```python
from build123d import *

# Parameters (mm, degrees)
BOSS_EXTRUDE2_DEPTH = 6.35
SKETCH4_R           = 1.5
CUT_EXTRUDE1_DEPTH  = 6.35
SKETCH5_R           = 1.25
SKETCH5_W           = 6.35
SKETCH5_H           = 19.05
CUT_EXTRUDE2_DEPTH  = 6.35
SKETCH6_R           = 1.5
CUT_EXTRUDE3_DEPTH  = 6.35
SKETCH7_R           = 1.5
SKETCH7_W           = 6.35
SKETCH7_H           = 19.05
CUT_EXTRUDE4_DEPTH  = 6.35
SKETCH9_R           = 1.5
CUT_EXTRUDE6_DEPTH  = 6.35
SKETCH10_R          = 1.5
CUT_EXTRUDE7_DEPTH  = 7.35


with BuildPart() as part:
    # Sketch3 → Boss-Extrude2 (new body)
    with BuildSketch(Plane(origin=(0, 0, 0), x_dir=(1, 0, 0), z_dir=(0, 1, 0))):
        with BuildLine():
            Line((-156.21, -76.2), (156.21, -76.2))
            ThreePointArc((156.21, -76.2), (174.170512242, -68.760512242), (181.61, -50.8))
            Line((181.61, -50.8), (181.61, 50.8))
            ThreePointArc((181.61, 50.8), (174.170512242, 68.760512242), (156.21, 76.2))
            Line((156.21, 76.2), (-156.21, 76.2))
            ThreePointArc((-156.21, 76.2), (-174.170512242, 68.760512242), (-181.61, 50.8))
            Line((-181.61, 50.8), (-181.61, -50.8))
            ThreePointArc((-181.61, -50.8), (-174.170512242, -68.760512242), (-156.21, -76.2))
        make_face()
    extrude(amount=-BOSS_EXTRUDE2_DEPTH)

    # Sketch4 → Cut-Extrude1 (cut)
    with BuildSketch(Plane(origin=(0, 0, 0), x_dir=(1, 0, 0), z_dir=(0, 1, 0))):
        with Locations((-44.45, 59.944)):
            Circle(SKETCH4_R)
        with Locations((69.85, 59.944)):
            Circle(SKETCH4_R)
        with Locations((69.85, -54.356)):
            Circle(SKETCH4_R)
        with Locations((-44.45, -54.356)):
            Circle(SKETCH4_R)
        with Locations((139.446, 20.066)):
            Circle(SKETCH4_R)
        with Locations((101.854, -17.526)):
            Circle(SKETCH4_R)
    extrude(amount=-CUT_EXTRUDE1_DEPTH, mode=Mode.SUBTRACT)

    # Sketch5 → Cut-Extrude2 (cut)
    with BuildSketch(Plane(origin=(0, 0, 0), x_dir=(1, 0, 0), z_dir=(0, 1, 0))):
        with Locations((-149.479, 15.875)):
            Circle(SKETCH5_R)
        with Locations((-149.479, -15.875)):
            Circle(SKETCH5_R)
        with Locations((-66.929, -15.875)):
            Circle(SKETCH5_R)
        with Locations((-66.929, 15.875)):
            Circle(SKETCH5_R)
        with Locations((-149.479, 0)):
            Rectangle(SKETCH5_W, SKETCH5_H)
        with Locations((-66.929, 0)):
            Rectangle(SKETCH5_W, SKETCH5_H)
    extrude(amount=-CUT_EXTRUDE2_DEPTH, mode=Mode.SUBTRACT)

    # Sketch6 → Cut-Extrude3 (cut)
    with BuildSketch(Plane(origin=(0, 0, 0), x_dir=(1, 0, 0), z_dir=(0, 1, 0))):
        with Locations((-157.988, 15.875)):
            Circle(SKETCH6_R)
        with Locations((-157.988, -15.875)):
            Circle(SKETCH6_R)
        with Locations((165.862, -15.875)):
            Circle(SKETCH6_R)
        with Locations((165.862, 15.875)):
            Circle(SKETCH6_R)
    extrude(amount=-CUT_EXTRUDE3_DEPTH, mode=Mode.SUBTRACT)

    # Sketch7 → Cut-Extrude4 (cut)
    with BuildSketch(Plane(origin=(0, 0, 0), x_dir=(1, 0, 0), z_dir=(0, 1, 0))):
        with Locations((-54.229, -28.575)):
            Circle(SKETCH7_R)
        with Locations((-54.229, -60.325)):
            Circle(SKETCH7_R)
        with Locations((99.441, -60.325)):
            Circle(SKETCH7_R)
        with Locations((99.441, -28.575)):
            Circle(SKETCH7_R)
        with Locations((99.441, -44.45)):
            Rectangle(SKETCH7_W, SKETCH7_H)
        with Locations((-54.229, -44.45)):
            Rectangle(SKETCH7_W, SKETCH7_H)
    extrude(amount=-CUT_EXTRUDE4_DEPTH, mode=Mode.SUBTRACT)

    # Sketch9 → Cut-Extrude6 (cut)
    with BuildSketch(Plane(origin=(0, 0, 0), x_dir=(1, 0, 0), z_dir=(0, 1, 0))):
        with Locations((-108.204, -71.12)):
            Circle(SKETCH9_R)
        with Locations((14.732, -71.12)):
            Circle(SKETCH9_R)
        with Locations((35.306, -71.12)):
            Circle(SKETCH9_R)
    extrude(amount=-CUT_EXTRUDE6_DEPTH, mode=Mode.SUBTRACT)

    # Sketch10 → Cut-Extrude7 (cut, through all)
    with BuildSketch(Plane(origin=(0, 0, 0), x_dir=(1, 0, 0), z_dir=(0, 1, 0))):
        with Locations((-124.61, 28.5)):
            Circle(SKETCH10_R)
        with Locations((-124.61, -28.5)):
            Circle(SKETCH10_R)
    extrude(amount=-CUT_EXTRUDE7_DEPTH, mode=Mode.SUBTRACT)


solid = part.part
```
Input: part model. Units: mm. Frame: model coordinates. A direction names the side the tool comes from. Give positions to 0.01 mm unless a question says otherwise; leave off trailing zeros. Order: outer loops, then holes, each group sorted by start corner. A loop starts at its lowest first (then second) coordinate and runs counter-clockwise, first axis right, second up. Notation, with made-up numbers: M 45.5,62.25 L 80.5,62.25 A30 cw 80.5,92.25 Z; hole C -16,53 d10. An arc over 180 degrees is marked long. Return JSON: item names as keys, results as strings.
1) Access query for faces 1 (the face through (-3, 0, -1)), 2 (the face through (-146.304, -3, 0)). Directions: +Z, -Z, +X, -X, +Y, -Y. A direction counts if a zero-diameter tool reaches every point of the face in a straight line with its end or side. Return the directions, or none.
Taken from the geometry:
{"face 1": "+Z, -Z, +X, -X, +Y", "face 2": "+Y, -Y"}
2) Section query B-B on y = -3. Count the separate pieces of the cut face and the enclosed holes in it, and give its area (3 significant figures).
Taken from the geometry:
{"separate pieces": "1", "enclosed holes": "27", "area": "54,200 mm2"}
3) Contact query for flat-ended pins moving along their axis: pin 1 (3.5 mm diameter, centred on x = -54.229, z = 28.575, fed in from -Y); pin 2 (2 mm diameter, centred on y = -5.5, z = -56, fed in from -X). Output: stop coordinate, or through.
Taken from the geometry:
{"pin 1": "stops at y = -6.35", "pin 2": "stops at x = -181.26"}
4) Line query: L1, parallel to X at y = -2, z = -7; L2, parallel to Z at x = 69.85, y = -1.25; L3, parallel to X at y = -1.75, z = 44. Output: solid intervals per line, ascending. Write a range as [from, to].
Taken from the geometry:
{"L1": "x = [-181.61, -152.65], [-146.3, -70.1], [-63.75, 181.61]", "L2": "z = [-76.2, -61.44], [-58.44, 52.86], [55.86, 76.2]", "L3": "x = [-181.61, -57.4], [-51.05, 96.27], [102.62, 181.61]"}
5) Mould query, pull axis Z, two halves, no side actions, for faces 3 (the face through (2, -3, -76.2)), 4 (the face through (173.97, -3.13, 68.96)), 5 (the face through (-150, -3, -9.525)). Classes: released by +Z, released by -Z, zero draft, split by the parting line, or undercut.
Taken from the geometry:
{"face 3": "released by -Z", "face 4": "released by +Z", "face 5": "undercut"}
6) Section query A-A on z = 5.5. Output: boundary loops of the cut face in (x, y).
Taken from the geometry:
{"outline": "M -181.61,-6.35 L -152.65,-6.35 L -152.65,0 L -181.61,0 Z; M -146.3,-6.35 L -70.1,-6.35 L -70.1,0 L -146.3,0 Z; M -63.75,-6.35 L 181.61,-6.35 L 181.61,0 L -63.75,0 Z"}
